```python
from build123d import *

# Parameters (mm, degrees)
SKETCH1_R           = 50
BOSS_EXTRUDE1_DEPTH = 50
BOSS_EXTRUDE2_REACH = 202
SKETCH2_R           = 45


with BuildPart() as part:
    # Sketch1 → Boss-Extrude1 (new body, symmetric)
    with BuildSketch(Plane.XY):
        with BuildLine():
            Line((-80, -40), (-80, 40))
            Line((-80, 40), (-22.281665693, 61.061668614))
            ThreePointArc((-22.281665693, 61.061668614), (65, 0), (-22.281665693, -61.061668614))
            Line((-22.281665693, -61.061668614), (-80, -40))
        make_face()
        Circle(SKETCH1_R, mode=Mode.SUBTRACT)
    extrude(amount=BOSS_EXTRUDE1_DEPTH, both=True)

    # Sketch2 → Boss-Extrude2 (add, up to next)
    with BuildSketch(Plane(origin=(120, 0, 0), x_dir=(0, 0, -1), z_dir=(1, 0, 0)), mode=Mode.PRIVATE) as boss_extrude2_sk1:
        Circle(SKETCH2_R)
    boss_extrude2_tool1 = extrude(boss_extrude2_sk1.sketch, amount=-BOSS_EXTRUDE2_REACH, mode=Mode.PRIVATE) - part.part
    add(boss_extrude2_tool1.solids().sort_by_distance((120, 0, 0))[0])

    # Sketch4 → Revolve1 (revolve)
    with BuildSketch(Plane.XY):
        Polygon((120, 0), (120, -20), (134, -20), (134, -25), (149, -25), (149, -15), (158.653629462, -12.390893217), (158.653629462, -6.923969146), (195, 0), align=None)
    revolve(axis=Axis((0, 0, 0), (1, 0, 0)))


solid = part.part
```
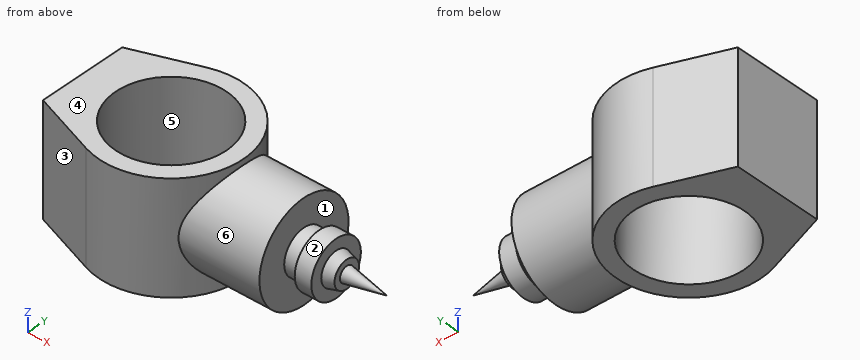
Work out the finished part from the listing and answer in its coordinate system (mm). Face numbers are marked on the shaded views. A direction names the side the tool comes from. Coordinates: 2 decimals unless noted, no trailing zeros. Order: outer loops, then holes, each group sorted by start corner. A loop starts at its lowest first (then second) coordinate and runs counter-clockwise, first axis right, second up. Notation, with made-up numbers: (10, 24) - (23, 24) arc R16 cw to (23, 47) - close; hole circle Ø3 at (11.5, 49.25). An arc over 180 degrees is marked (long way). Answer as a JSON object with one key per item and string values.
1. Each of these flat-tipped pins is pushed along its axis until it touches: P1, Ø8, axis at y = -33.5, z = 14.5, coming from the +X side; P2, Ø10, axis at x = 123, z = -14, coming from the -Y side; P3, Ø1, axis at x = 76.5, y = -18, coming from the +Z side. Where does it stop, or does it pass through?
Output values:
{"P1": "stops at x = 120", "P2": "stops at y = -43.87", "P3": "stops at z = 41.46"}
2. Consider line 1 (Y direction, x = 0, z = -25); line 2 (X direction, y = -20, z = -17); line 3 (X direction, y = 30, z = -26.5). Determine where each line is inside the solid, lowest interval first.
Output values:
{"line 1": "y = -65 to -50, 50 to 65", "line 2": "x = -80 to -45.83, 45.83 to 120", "line 3": "x = -80 to -40, 40 to 120"}
3. Find section A-A on x = 0. Determine the outline of the cut face in (y, z).
Output values:
{"outline": "(-65, -50) - (-50, -50) - (-50, 50) - (-65, 50) - close; (50, -50) - (65, -50) - (65, 50) - (50, 50) - close"}
4. Find section B-B on z = 40. Determine the outline of the cut face in (x, y), plus the area to 3 significant figures.
Output values:
{"outline": "(-80, -40) - (-22.28, -61.06) arc R65 ccw to (61.64, -20.62) - (120, -20.62) - (120, 20.62) - (61.64, 20.62) arc R65 ccw to (-22.28, 61.06) - (-80, 40) - close; hole circle Ø100 at (0, 0)", "area": "9,770 mm²"}
5. Find section D-D on x = -60. Determine the outline of the cut face in (y, z).
Output values:
{"outline": "(-47.3, -50) - (47.3, -50) - (47.3, 50) - (-47.3, 50) - close"}
6. A tool of negligible diameter and unlimited length cuts with its end or side. For the marked faces 1, 2 and 3, from which of +Z, -Z, +X, -X, +Y, -Y can it reach the whole face along a straight path? Write none if from no direction.
Output values:
{"face 1": "none", "face 2": "+X", "face 3": "+Z, -Z, -X, -Y"}
7. Find section C-C on x = 70. Determine the outline of the cut face in (y, z).
Output values:
{"outline": "circle Ø90 at (0, 0)"}
8. The mould has two halves that part along Y. Classify the marked faces 4, 5 and 6: +Y half, -Y half, draft (parallel to the pull), parting line (faces both ways), or undercut.
Output values:
{"face 4": "draft", "face 5": "undercut", "face 6": "parting line"}
